from build123d import *

# Parameters (mm, degrees)
F0_W      = 15
F0_H      = 15
F1_DEPTH  = 25
F2_W      = 9
F2_H      = 9
F3_DEPTH  = 23
F6_DEPTH  = 15.001
F8_DEPTH  = 15.001
F9_W      = 15
F9_H      = 15
F9_W_2    = 13
F9_H_2    = 13
F10_DEPTH = 40.4


with BuildPart() as f1:
    # F0 (on Top) → F1 (new body)
    with BuildSketch(Plane.XY):
        Rectangle(F0_W, F0_H)
    extrude(amount=F1_DEPTH)

    # F2 (on face) → F3 (cut)
    with BuildSketch(Plane.XY.offset(25)):
        Rectangle(F2_W, F2_H)
    extrude(amount=-F3_DEPTH, mode=Mode.SUBTRACT)

    # F5 (on face) → F6 (cut, through all)
    with BuildSketch(Plane.XZ.offset(7.5)):
        Polygon((3.5, 25), (-3.5, 25), (0, 14.5), align=None)
        Polygon((0, 12.5), (-3.5, 2), (3.5, 2), align=None)
        Polygon((-1, 13.5), (-4.5, 24), (-4.5, 3), align=None)
        Polygon((4.5, 3), (4.5, 24), (1, 13.5), align=None)
    extrude(amount=-F6_DEPTH, mode=Mode.SUBTRACT)

    # F7 (on face) → F8 (cut, through all)
    with BuildSketch(Plane.YZ.offset(7.5)):
        Polygon((3.5, 25), (-3.5, 25), (0, 14.5), align=None)
        Polygon((0, 12.5), (-3.5, 2), (3.5, 2), align=None)
        Polygon((4.5, 3), (4.5, 24), (1, 13.5), align=None)
        Polygon((-1, 13.5), (-4.5, 24), (-4.5, 3), align=None)
    extrude(amount=-F8_DEPTH, mode=Mode.SUBTRACT)

    # F9 (on face) → F10 (cut)
    with BuildSketch(Plane.XY.offset(2)):
        Rectangle(F9_W, F9_H)
        Rectangle(F9_W_2, F9_H_2, mode=Mode.SUBTRACT)
    extrude(amount=F10_DEPTH, mode=Mode.SUBTRACT)


solid = f1.part
Source: CAD feature listing. Evaluate the final solid. Frame: model axes, mm. A direction names the side the tool comes from. Give positions to 0.01 mm unless a question says otherwise; leave off trailing zeros. Loops run counter-clockwise (first coordinate to the right, second up) from the corner with the lowest first, then second, coordinate; pieces in that order, holes last. Notation, with made-up numbers: (86, 73.5) -> (121, 73.5) arc R25 cw to (121, 98.5) -> close; hole circle Ø8 at (88, 10.25). An arc over 180 degrees is marked (long way). Use a Markdown table: item, result. Add a question column.
1) Line query: line 1 along X through (y, z) = (-6.25, 13.5); line 2 along Y through (x, z) = (6, 22.5); line 3 along Y through (x, z) = (1.25, 15). Output: solid intervals per line, ascending. Write a range as [from, to].
2) Pull-direction query (Z, two-part tool) for faces 1 (the face through (7.5, 0, 1)), 2 (the face through (0, 0, 0)), 3 (the face through (-5.486, -2.726, 18.676)); classes: +Z half, -Z half, draft (parallel to the pull), parting line (faces both ways), or undercut.
3) Section query D-D, the plane z = 13. Count the separate pieces of the cut face and the enclosed holes in it, then the cut area to 3 significant figures.
4) Section query C-C, the plane y = -3. Return the cut outline in (x, z).
5) First-contact query: pin 1 (6 mm diameter, centred on x = 3, z = 15.5, fed in from -Y); pin 2 (6.5 mm diameter, centred on y = 2.5, z = 18, fed in from -X); pin 3 (1 mm diameter, centred on y = -6, z = 17.5, fed in from +X). Flat tips, straight axial feed; report the tip coordinate or a pass-through.
6) Reachability of faces 4 (the face through (-1.774, -5.514, 19.824)), 5 (the face through (-1.726, -5.514, 7.323)), 6 (the face through (-5.486, -1.774, 19.824)) from +Z, -Z, +X, -X, +Y, -Y: full face, straight path, thin tool, end or side. Return the list, or none.
7) Section query B-B, the plane x = -1.75. Return the cut outline in (y, z).
8) Section query A-A, the plane y = 5.25. Return the cut outline in (x, z), then the cut area to 3 significant figures.
Numbers:
| question | item | result |
|---|---|---|
| 1 | line 1 | x = [-6.5, -4.5], [-1, 1], [4.5, 6.5] |
| 1 | line 2 | y = [-6.5, -4.5], [-4, -2.67], [2.67, 4], [4.5, 6.5] |
| 1 | line 3 | y = [-6.5, -4.5], [4.5, 6.5] |
| 2 | face 1 | draft |
| 2 | face 2 | -Z half |
| 2 | face 3 | undercut |
| 3 | separate pieces | 8 |
| 3 | enclosed holes | 0 |
| 3 | area | 34.7 mm2 |
| 4 | outline | (-7.5, 0) -> (7.5, 0) -> (7.5, 2) -> (-7.5, 2) -> close; (-6.5, 3.5) -> (-4.5, 3.5) -> (-4.5, 7.5) -> (-6.5, 7.5) -> close; (-6.5, 19.5) -> (-4.5, 19.5) -> (-4.5, 23.5) -> (-6.5, 23.5) -> close; (4.5, 3.5) -> (6.5, 3.5) -> (6.5, 7.5) -> (4.5, 7.5) -> close; (4.5, 19.5) -> (6.5, 19.5) -> (6.5, 23.5) -> (4.5, 23.5) -> close |
| 5 | pin 1 | stops at y = -6.5 |
| 5 | pin 2 | stops at x = -6.5 |
| 5 | pin 3 | stops at x = 6.5 |
| 6 | face 4 | +Z, +Y, -Y |
| 6 | face 5 | +Y, -Y |
| 6 | face 6 | +Z, +X, -X |
| 7 | outline | (-7.5, 0) -> (7.5, 0) -> (7.5, 2) -> (-7.5, 2) -> close; (-6.5, 7.25) -> (-4.5, 7.25) -> (-4.5, 11.25) -> (-6.5, 11.25) -> close; (-6.5, 15.75) -> (-4.5, 15.75) -> (-4.5, 19.75) -> (-6.5, 19.75) -> close; (4.5, 7.25) -> (6.5, 7.25) -> (6.5, 11.25) -> (4.5, 11.25) -> close; (4.5, 15.75) -> (6.5, 15.75) -> (6.5, 19.75) -> (4.5, 19.75) -> close |
| 8 | outline | (-7.5, 0) -> (7.5, 0) -> (7.5, 2) -> (6.5, 2) -> (6.5, 25) -> (3.5, 25) -> (0, 14.5) -> (-3.5, 25) -> (-6.5, 25) -> (-6.5, 2) -> (-7.5, 2) -> close; hole (-4.5, 3) -> (-1, 13.5) -> (-4.5, 24) -> close; hole (-3.5, 2) -> (3.5, 2) -> (0, 12.5) -> close; hole (1, 13.5) -> (4.5, 3) -> (4.5, 24) -> close |
| 8 | area | 182 mm2 |
